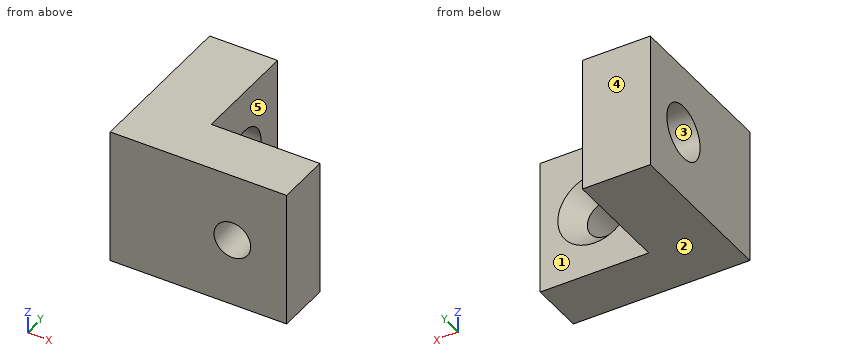
```python
from build123d import *

# Parameters (mm, degrees)
SKETCH1_W                                       = 40
SKETCH1_H                                       = 50
BOSS_EXTRUDE1_DEPTH                             = 20
CSK_FOR_M2_FLAT_HEAD_MACHINE_SCREW1_D           = 13.5
CSK_FOR_M2_FLAT_HEAD_MACHINE_SCREW1_CSINK_D     = 27
CSK_FOR_M2_FLAT_HEAD_MACHINE_SCREW1_CSINK_ANGLE = 90
SKETCH4_W                                       = 50
SKETCH4_H                                       = 60
SKETCH4_R                                       = 10
BOSS_EXTRUDE2_DEPTH                             = 25


with BuildPart() as part:
    # Sketch1 → Boss-Extrude1 (new body)
    with BuildSketch(Plane(origin=(0, 0, 0), x_dir=(1, 0, 0), z_dir=(0, 1, 0))):
        with Locations((20, -25)):
            Rectangle(SKETCH1_W, SKETCH1_H)
    extrude(amount=BOSS_EXTRUDE1_DEPTH)

    # CSK for M2 Flat Head Machine Screw1 (through all)
    with Locations(Plane(origin=(0, 20, 0), x_dir=(1, 0, 0), z_dir=(0, 1, 0))):
        with Locations((20, -25)):
            CounterSinkHole(CSK_FOR_M2_FLAT_HEAD_MACHINE_SCREW1_D / 2, CSK_FOR_M2_FLAT_HEAD_MACHINE_SCREW1_CSINK_D / 2, counter_sink_angle=CSK_FOR_M2_FLAT_HEAD_MACHINE_SCREW1_CSINK_ANGLE)

    # Sketch4 → Boss-Extrude2 (add)
    with BuildSketch(Plane.ZY):
        with Locations((25, 30)):
            Rectangle(SKETCH4_W, SKETCH4_H)
        with Locations((25, 40)):
            Circle(SKETCH4_R, mode=Mode.SUBTRACT)
    extrude(amount=BOSS_EXTRUDE2_DEPTH)


solid = part.part
```
Input: part model. Units: mm. Frame: model coordinates. Face numbers are marked on the shaded views. A direction names the side the tool comes from. Give positions to 0.01 mm unless a question says otherwise; leave off trailing zeros. Loops run counter-clockwise (first coordinate to the right, second up) from the corner with the lowest first, then second, coordinate; pieces in that order, holes last. Notation, with made-up numbers: M 41,74 L 78,74 A24 cw 78,97 Z; hole C 21,-0.5 d6. An arc over 180 degrees is marked long. Answer as CSV lines item,"result". Start each with the question number.
1. Section B-B on x = 20. Return loops of the section in (y, z), plus the area to 3 significant figures.
2. Line query: L1, parallel to Y at x = -7, z = 25; L2, parallel to X at y = 4, z = 25; L3, parallel to X at y = 31.5, z = 2. Output: solid intervals per line, ascending.
3. Reachability of the marked faces 1 and 2 from +Z, -Z, +X, -X, +Y, -Y: full face, straight path, thin tool, end or side. Return the list, or none.
4. Section C-C on y = 10. Return loops of the section in (x, z).
5. Section A-A on y = 40. Return loops of the section in (x, z), plus the area to 3 significant figures.
6. Pin query (flat end, axial travel): P1, Ø3, axis at y = 45, z = 34.5, coming from the +X side; P2, Ø1.5, axis at x = 32.5, z = 14.5, coming from the +Y side. Return the tip coordinate at first contact, or that it passes through.
7. Section D-D on z = 44. Return loops of the section in (x, y).
8. Pull-direction query (Y, two-part tool) for the marked faces 3, 4 and 5; classes: released by +Y, released by -Y, zero draft, split by the parting line, or undercut.
Computed values:
1,outline,"M 0,0 L 20,0 L 20,11.5 L 13.25,18.25 L 0,18.25 Z; M 0,31.75 L 13.25,31.75 L 20,38.5 L 20,50 L 0,50 Z"
1,area,"684 mm²"
2,L1,"y = 0 to 30, 50 to 60"
2,L2,"x = -25 to 13.25, 26.75 to 40"
2,L3,"x = -25 to 0"
3,face 1,"+Z, -Z, +X, +Y"
3,face 2,"-Z, +X, -X, +Y, -Y"
4,outline,"M -25,0 L 40,0 L 40,50 L -25,50 Z; hole C 20,25 d13.5"
5,outline,"M -25,0 L 0,0 L 0,15 L -25,15 Z; M -25,35 L 0,35 L 0,50 L -25,50 Z"
5,area,"750 mm²"
6,P1,"stops at x = 0"
6,P2,"stops at y = 20"
7,outline,"M -25,0 L 40,0 L 40,20 L 0,20 L 0,60 L -25,60 Z"
8,face 3,"undercut"
8,face 4,"released by +Y"
8,face 5,"zero draft"
